Verification items for the finished model (mm, model axes). Face numbers are marked on the shaded views. A direction names the side the tool comes from. Coordinates: 2 decimals unless noted, no trailing zeros. Write each loop counter-clockwise with the first axis right and the second up, starting at its lowest first coordinate (ties: lowest second). Pieces come first, ordered by that corner, then holes. Notation, with made-up numbers: (67.25, -14.5) -> (91.25, -14.5) arc R15 cw to (91.25, 2.5) -> close; hole circle Ø6 at (-5.5, 8). An arc over 180 degrees is marked (long way). Answer in a Markdown table with one row per item.
```python
from build123d import *

# Parameters (mm, degrees)
SKETCH1_W           = 50
SKETCH1_H           = 21
BOSS_EXTRUDE1_DEPTH = 58
SKETCH3_R           = 7.5
CUT_EXTRUDE1_DEPTH  = 24
CUT_EXTRUDE2_REACH  = 66.025
SKETCH4_R           = 5
CUT_EXTRUDE3_START  = -24
SKETCH5_R           = 7.5
CUT_EXTRUDE3_DEPTH  = 24
CUT_EXTRUDE4_REACH  = 66.025
SKETCH6_R           = 4.5
CUT_EXTRUDE5_REACH  = 68.558
SKETCH8_W           = 10
SKETCH8_H           = 18
SKETCH9_W           = 5
SKETCH9_H           = 58
BOSS_EXTRUDE3_DEPTH = 48
CUT_EXTRUDE7_REACH  = 95.916
BOSS_EXTRUDE4_DEPTH = 4
FILLET1_R           = 5
SKETCH7_R           = 4.1
CUT_EXTRUDE8_DEPTH  = 15


with BuildPart() as part:
    # Sketch1 → Boss-Extrude1 (new body)
    with BuildSketch(Plane(origin=(0, 0, 0), x_dir=(1, 0, 0), z_dir=(0, 1, 0))):
        Rectangle(SKETCH1_W, SKETCH1_H)
    extrude(amount=BOSS_EXTRUDE1_DEPTH)

    # Sketch3 → Cut-Extrude1 (cut)
    with BuildSketch(Plane(origin=(0, 58, 0), x_dir=(1, 0, 0), z_dir=(0, 1, 0))):
        with Locations(Location((-15, 0, 0), (0, 0, 270))):
            Circle(SKETCH3_R)
    extrude(amount=-CUT_EXTRUDE1_DEPTH, mode=Mode.SUBTRACT)

    # Sketch4 → Cut-Extrude2 (cut, up to next)
    with BuildSketch(Plane(origin=(0, 58, 0), x_dir=(1, 0, 0), z_dir=(0, 1, 0)), mode=Mode.PRIVATE) as cut_extrude2_sk1:
        with Locations(Location((15, 0, 0), (0, 0, 270))):
            Circle(SKETCH4_R)
    cut_extrude2_tool1 = extrude(cut_extrude2_sk1.sketch, amount=-CUT_EXTRUDE2_REACH, mode=Mode.PRIVATE) & part.part
    add(cut_extrude2_tool1.solids().sort_by_distance((15, 58, 0))[0], mode=Mode.SUBTRACT)

    # Sketch5 → Cut-Extrude3 (cut)
    with BuildSketch(Plane.XZ.offset(CUT_EXTRUDE3_START)):
        with Locations(Location((-15, 0, 0), (0, 0, 90))):
            Circle(SKETCH5_R)
    extrude(amount=CUT_EXTRUDE3_DEPTH, mode=Mode.SUBTRACT)

    # Sketch6 → Cut-Extrude4 (cut, up to next)
    with BuildSketch(Plane.XZ, mode=Mode.PRIVATE) as cut_extrude4_sk1:
        with Locations(Location((-15, 0, 0), (0, 0, 270))):
            Circle(SKETCH6_R)
    cut_extrude4_tool1 = extrude(cut_extrude4_sk1.sketch, amount=-CUT_EXTRUDE4_REACH, mode=Mode.PRIVATE) & part.part
    add(cut_extrude4_tool1.solids().sort_by_distance((-15, 0, 0))[0], mode=Mode.SUBTRACT)

    # Sketch8 → Cut-Extrude5 (cut, up to next)
    with BuildSketch(Plane.XY.offset(10.5), mode=Mode.PRIVATE) as cut_extrude5_sk1:
        with Locations((0, 29)):
            Rectangle(SKETCH8_W, SKETCH8_H)
    cut_extrude5_tool1 = extrude(cut_extrude5_sk1.sketch, amount=-CUT_EXTRUDE5_REACH, mode=Mode.PRIVATE) & part.part
    add(cut_extrude5_tool1.solids().sort_by_distance((0, 29, 10.5))[0], mode=Mode.SUBTRACT)

    # Sketch9 → Boss-Extrude3 (add)
    with BuildSketch(Plane(origin=(0, 0, -10.5), x_dir=(-1, 0, 0), z_dir=(0, 0, -1))):
        with Locations((17.6, 29)):
            Rectangle(SKETCH9_W, SKETCH9_H)
    extrude(amount=BOSS_EXTRUDE3_DEPTH)

    # Sketch10 → Cut-Extrude7 (cut, up to next)
    with BuildSketch(Plane.ZY.offset(20.1), mode=Mode.PRIVATE) as cut_extrude7_sk1:
        with BuildLine():
            Line((-41.5, 17), (-27.5, 17))
            ThreePointArc((-27.5, 17), (-23.964466094, 18.464466094), (-22.5, 22))
            Line((-22.5, 22), (-22.5, 36))
            ThreePointArc((-22.5, 36), (-23.964466094, 39.535533906), (-27.5, 41))
            Line((-27.5, 41), (-41.5, 41))
            ThreePointArc((-41.5, 41), (-45.035533906, 39.535533906), (-46.5, 36))
            Line((-46.5, 36), (-46.5, 22))
            ThreePointArc((-46.5, 22), (-45.035533906, 18.464466094), (-41.5, 17))
        make_face()
    cut_extrude7_tool1 = extrude(cut_extrude7_sk1.sketch, amount=-CUT_EXTRUDE7_REACH, mode=Mode.PRIVATE) & part.part
    # Sketch10 → Cut-Extrude7 (cut, up to next)
    with BuildSketch(Plane.ZY.offset(20.1), mode=Mode.PRIVATE) as cut_extrude7_sk2:
        with BuildLine():
            Line((-15.5, 42.7), (-53.5, 42.7))
            ThreePointArc((-53.5, 42.7), (-55.25, 44.45), (-53.5, 46.2))
            Line((-53.5, 46.2), (-15.5, 46.2))
            ThreePointArc((-15.5, 46.2), (-13.75, 44.45), (-15.5, 42.7))
        make_face()
    cut_extrude7_tool2 = extrude(cut_extrude7_sk2.sketch, amount=-CUT_EXTRUDE7_REACH, mode=Mode.PRIVATE) & part.part
    # Sketch10 → Cut-Extrude7 (cut, up to next)
    with BuildSketch(Plane.ZY.offset(20.1), mode=Mode.PRIVATE) as cut_extrude7_sk3:
        with BuildLine():
            Line((-15.5, 15.3), (-53.5, 15.3))
            ThreePointArc((-53.5, 15.3), (-55.25, 13.55), (-53.5, 11.8))
            Line((-53.5, 11.8), (-15.5, 11.8))
            ThreePointArc((-15.5, 11.8), (-13.75, 13.55), (-15.5, 15.3))
        make_face()
    cut_extrude7_tool3 = extrude(cut_extrude7_sk3.sketch, amount=-CUT_EXTRUDE7_REACH, mode=Mode.PRIVATE) & part.part
    add(cut_extrude7_tool1.solids().sort_by_distance((-20.1, 29, -34.5))[0], mode=Mode.SUBTRACT)
    add(cut_extrude7_tool2.solids().sort_by_distance((-20.1, 44.45, -34.5))[0], mode=Mode.SUBTRACT)
    add(cut_extrude7_tool3.solids().sort_by_distance((-20.1, 13.55, -34.5))[0], mode=Mode.SUBTRACT)

    # Sketch11 → Boss-Extrude4 (add)
    with BuildSketch(Plane(origin=(0, 0, 0), x_dir=(-1, 0, 0), z_dir=(0, -1, 0))):
        Polygon((15.1, 58.5), (-25, 10.5), (15.1, 10.5), align=None)
        Polygon((20.1, 58.5), (20.1, 10.5), (25, 10.5), align=None)
    boss_extrude4 = extrude(amount=-BOSS_EXTRUDE4_DEPTH)

    # Mirror1: Boss-Extrude4 across plane
    add(boss_extrude4.mirror(Plane(origin=(0, 29, 0), x_dir=(0, 0, 1), z_dir=(0, -1, 0))))

    # Fillet1
    fillet1_edges = [part.edges().sort_by_distance(p)[0] for p in [
        (25, 29, 10.5),
        (-25, 29, 10.5),
    ]]
    fillet(fillet1_edges, radius=FILLET1_R)

    # Sketch7 → Cut-Extrude8 (cut)
    with BuildSketch(Plane.XY.offset(10.5)):
        with Locations((0, 46)):
            Circle(SKETCH7_R)
        with Locations(Location((0, 12, 0), (0, 0, 180))):
            Circle(SKETCH7_R)
    extrude(amount=-CUT_EXTRUDE8_DEPTH, mode=Mode.SUBTRACT)


solid = part.part
```
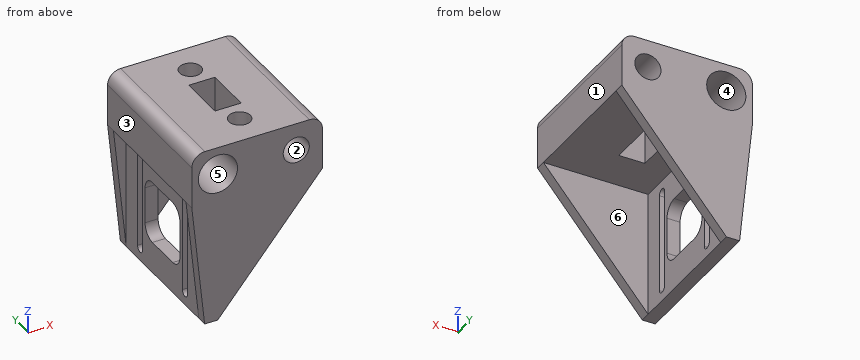
1. Depth check by flat-ended pin: P1, Ø24, axis at y = 28.5, z = -35.5, coming from the +X side; P2, Ø5, axis at x = 0, y = 46, coming from the +Z side; P3, Ø4, axis at x = -10.5, y = 28, coming from the -Z side. Enter the tip coordinate at first touch or a pass-through.
Geometry says:
| item | result |
|---|---|
| P1 | x = -15.1 |
| P2 | z = -4.5 |
| P3 | z = -10.5 |
2. Mould release check, pull along X, two halves, no side actions. Record for the marked faces 1, 2 and 3: released by +X, released by -X, zero draft, split by the parting line, or undercut.
Geometry says:
| item | result |
|---|---|
| face 1 | released by +X |
| face 2 | undercut |
| face 3 | released by -X |
3. Section check C-C, the plane x = 15. Record the boundary of the cut face in (y, z), plus the area to 3 significant figures.
Geometry says:
| item | result |
|---|---|
| outline | (0, -22.47) -> (4, -22.47) -> (4, -10.5) -> (54, -10.5) -> (54, -22.47) -> (58, -22.47) -> (58, -5) -> (0, -5) -> close; (0, 5) -> (58, 5) -> (58, 10.5) -> (0, 10.5) -> close |
| area | 734 mm^2 |
4. Thickness scan on line 1 (X direction, y = 22, z = 0); line 2 (Y direction, x = 0, z = -1); line 3 (X direction, y = 11.75, z = 0). Record the ranges inside material, lowest first. Write a range as from..to.
Geometry says:
| item | result |
|---|---|
| line 1 | -25..-22.5, -7.5..-5, 5..10, 20..25 |
| line 2 | 0..7.9, 16.1..20, 38..41.9, 50.1..58 |
| line 3 | -25..-22.5, -7.5..-4.09, 4.09..10, 20..25 |
5. Section check D-D, the plane y = 51. Record the boundary of the cut face in (x, z), plus the area to 3 significant figures.
Geometry says:
| item | result |
|---|---|
| outline | (-25, -10.5) -> (-20.1, -10.5) -> (-20.1, -58.5) -> (-15.1, -58.5) -> (-15.1, -10.5) -> (25, -10.5) -> (25, 5.5) arc R5 ccw to (20, 10.5) -> (-20, 10.5) arc R5 ccw to (-25, 5.5) -> close; hole circle Ø15 at (-15, 0); hole circle Ø10 at (15, 0) |
| area | 1,020 mm^2 |
6. Tool access check on the marked faces 4, 5 and 6. Record the directions out of +Z, -Z, +X, -X, +Y, -Y that give a thin tool (end or side, any length) a straight path to the whole face; none if there is none.
Geometry says:
| item | result |
|---|---|
| face 4 | +Y |
| face 5 | -Y |
| face 6 | -Z, +X |
7. Section check A-A, the plane y = 30. Record the boundary of the cut face in (x, z).
Geometry says:
| item | result |
|---|---|
| outline | (-25, -10.5) -> (-20.1, -10.5) -> (-20.1, -22.5) -> (-15.1, -22.5) -> (-15.1, -10.5) -> (-5, -10.5) -> (-5, 10.5) -> (-20, 10.5) arc R5 ccw to (-25, 5.5) -> close; (-20.1, -58.5) -> (-15.1, -58.5) -> (-15.1, -46.5) -> (-20.1, -46.5) -> close; (5, -10.5) -> (25, -10.5) -> (25, 5.5) arc R5 ccw to (20, 10.5) -> (5, 10.5) -> close; hole circle Ø9 at (-15, 0); hole circle Ø10 at (15, 0) |
8. Section check B-B, the plane z = 1. Record the boundary of the cut face in (x, y), plus the area to 3 significant figures.
Geometry says:
| item | result |
|---|---|
| outline | (-25, 0) -> (-22.43, 0) -> (-22.43, 24) -> (-19.39, 24) -> (-19.39, 34) -> (-22.43, 34) -> (-22.43, 58) -> (-25, 58) -> close; (-10.61, 24) -> (-7.57, 24) -> (-7.57, 0) -> (10.1, 0) -> (10.1, 58) -> (-7.57, 58) -> (-7.57, 34) -> (-10.61, 34) -> close; (19.9, 0) -> (25, 0) -> (25, 58) -> (19.9, 58) -> close; hole (-5, 20) -> (5, 20) -> (5, 38) -> (-5, 38) -> close; hole circle Ø8.2 at (0, 12); hole circle Ø8.2 at (0, 46) |
| area | 1,240 mm^2 |
